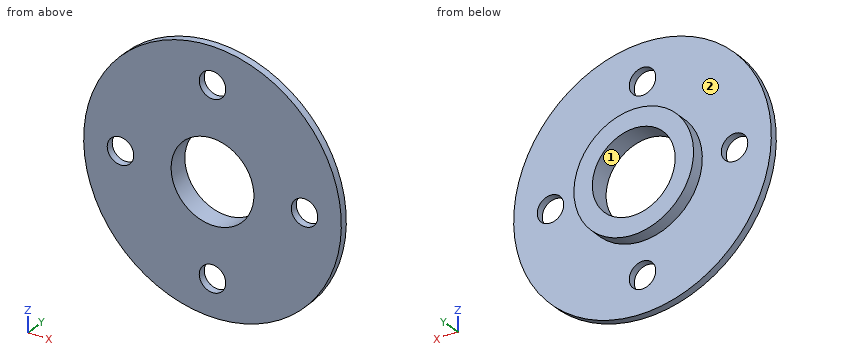
from build123d import *

# Parameters (mm, degrees)
F3_D = 28.575
F4_D = 9.144


with BuildPart() as f1:
    # F0 (on Right) → F1 (revolve)
    with BuildSketch(Plane.YZ):
        Polygon((0, 44.45), (0, 0), (6.985, 0), (6.985, 20.6375), (2.54, 20.6375), (2.54, 44.45), align=None)
    revolve(axis=Axis((0, 6.35, 0), (0, 1, 0)))

    # F3 (through all)
    with Locations(Plane.XZ):
        with Locations((0, 0)):
            Hole(F3_D / 2)

    # F4 (through all)
    with Locations(Plane.XZ):
        with Locations((0, 31.75), (31.75, 0), (0, -31.75), (-31.75, 0)):
            Hole(F4_D / 2)


solid = f1.part
Source: CAD feature listing. Evaluate the final solid. Frame: model axes, mm. Face numbers are marked on the shaded views. Coordinates: 2 decimals unless noted, no trailing zeros. Loops run counter-clockwise (first coordinate to the right, second up) from the corner with the lowest first, then second, coordinate; pieces in that order, holes last. Notation, with made-up numbers: (-14.5, -20) - (3.5, -20) arc R17 cw to (3.5, -10) - close; hole circle Ø4 at (57.25, 81). An arc over 180 degrees is marked (long way). Return JSON: item names as keys, results as strings.
Q1. Material intervals for line 1 along Z through (x, y) = (0.5, 3); line 2 along Y through (x, z) = (25, 20.5); line 3 along Z through (x, y) = (-28, 1.5), sorted ascending.
Results:
{"line 1": "-20.63 to -14.28, 14.28 to 20.63", "line 2": "0 to 2.54", "line 3": "-34.52 to -2.62, 2.62 to 34.52"}
Q2. Contact query for flat-ended pins moving along their axis: P1, Ø3, axis at y = 6, z = -7.5, coming from the -X side; P2, Ø1, axis at x = -2, y = 1, coming from the -Z side; P3, Ø2, axis at x = 16, y = 1, coming from the -Z side. Output: stop coordinate, or through.
Results:
{"P1": "x = -19.75", "P2": "z = -44.42", "P3": "z = -41.84"}
Q3. Section D-D, the plane z = 31.75. Return loops of the section in (x, y).
Results:
{"outline": "(-31.11, 0) - (-4.57, 0) - (-4.57, 2.54) - (-31.11, 2.54) - close; (4.57, 0) - (31.11, 0) - (31.11, 2.54) - (4.57, 2.54) - close"}
Q4. Section C-C, the plane x = -34.5. Return loops of the section in (y, z).
Results:
{"outline": "(0, -28.03) - (2.54, -28.03) - (2.54, -3.65) - (0, -3.65) - close; (0, 3.65) - (2.54, 3.65) - (2.54, 28.03) - (0, 28.03) - close"}
Q5. Mould query, pull axis Z, two halves, no side actions, for the marked faces 1 and 2. Classes: released by +Z, released by -Z, zero draft, split by the parting line, or undercut.
Results:
{"face 1": "undercut", "face 2": "zero draft"}
Q6. Section A-A, the plane z = 0. Give the number of separate pieces and of enclosed holes in the cut face, plus the area to 3 significant figures.
Results:
{"separate pieces": "4", "enclosed holes": "0", "area": "163 mm2"}
